from build123d import *

# Parameters (mm, degrees)
F0_W     = 76.2
F0_H     = 19.05
F0_W_2   = 19.05
F0_H_2   = 38.1
F0_R     = 17.4625
F0_W_3   = 20.17304
F1_DEPTH = 19.05
F0_R_2   = 6.35
F2_DEPTH = 9.525


with BuildPart() as f1:
    # F0 (on Front) → F1 (new body)
    with BuildSketch(Plane.XZ):
        Polygon((-489.430563, 76.2), (-540.230563, 76.2), (-540.230563, 95.25), (-591.030563, 95.25), (-599.913724, 95.25), (-613.971884, 125.397822), (-596.706721, 133.4487), (-618.175729, 179.489136), (-635.440892, 171.438258), (-656.9099, 217.478693), (-639.644736, 225.529571), (-661.113744, 271.570007), (-678.378907, 263.519129), (-699.847915, 309.559564), (-682.582752, 317.610442), (-704.051759, 363.650878), (-721.316923, 355.6), (-743.430563, 355.6), (-997.430563, 127), (-997.430563, 0), (-591.030563, 0), (342.419437, 0), (371.914191, 0), (392.43009, 43.996488), (447.893046, 162.937181), (502.200551, 162.937181), (676.493046, 162.937181), (676.493046, 239.137181), (676.493046, 258.187181), (624.570006, 258.187181), (624.570006, 239.137181), (573.770006, 239.137181), (573.770006, 258.187181), (522.970006, 258.187181), (522.970006, 239.137181), (472.170006, 239.137181), (472.170006, 258.187181), (421.370006, 258.187181), (421.370006, 239.137181), (399.256366, 239.137181), (381.991203, 247.188059), (360.522195, 201.147623), (377.787358, 193.096745), (356.318351, 147.05631), (339.053221, 155.107172), (317.579072, 109.055711), (334.844236, 101.004833), (323.369437, 76.2), (272.569437, 76.2), (272.569437, 95.25), (221.769437, 95.25), (221.769437, 76.2), (170.969437, 76.2), (170.969437, 95.25), (120.169437, 95.25), (120.169437, 76.2), (69.369437, 76.2), (69.369437, 95.25), (18.569437, 95.25), (18.569437, 76.2), (-32.230563, 76.2), (-32.230563, 95.25), (-83.030563, 95.25), (-83.030563, 76.2), (-133.830563, 76.2), (-133.830563, 95.25), (-184.630563, 95.25), (-184.630563, 76.2), (-235.430563, 76.2), (-235.430563, 95.25), (-286.230563, 95.25), (-286.230563, 76.2), (-337.030563, 76.2), (-337.030563, 95.25), (-387.830563, 95.25), (-387.830563, 76.2), (-438.630563, 76.2), (-438.630563, 95.25), (-489.430563, 95.25), align=None)
        with Locations((-705.330563, 34.925)):
            Rectangle(F0_W, F0_H, mode=Mode.SUBTRACT)
        with Locations((-581.505563, 44.45)):
            Rectangle(F0_W_2, F0_H_2, mode=Mode.SUBTRACT)
        with Locations((-932.085752, 57.15)):
            Circle(F0_R, mode=Mode.SUBTRACT)
        with Locations((-159.243268, 44.45)):
            Rectangle(F0_W_2, F0_H_2, mode=Mode.SUBTRACT)
        with Locations((351.944437, 44.45)):
            Rectangle(F0_W_2, F0_H_2, mode=Mode.SUBTRACT)
        Polygon((-832.288567, 215.839342), (-845.030563, 230.0007), (-788.385133, 280.968682), (-775.643137, 266.807325), align=None, mode=Mode.SUBTRACT)
        with Locations((411.845006, 201.037181)):
            Rectangle(F0_W_2, F0_H_2, mode=Mode.SUBTRACT)
        with Locations((549.493046, 191.512181)):
            Rectangle(F0_W, F0_H, mode=Mode.SUBTRACT)
        with Locations((641.006526, 201.037181)):
            Rectangle(F0_W_3, F0_H_2, mode=Mode.SUBTRACT)
    extrude(amount=-F1_DEPTH)

    # F0 (on Front) → F2 (join)
    with BuildSketch(Plane.XZ):
        with Locations((-932.085752, 57.15)):
            Circle(F0_R)
        with Locations((-932.085752, 57.15)):
            Circle(F0_R_2, mode=Mode.SUBTRACT)
    extrude(amount=-F2_DEPTH)


solid = f1.part
Part model, mm, in its own coordinate system. A direction names the side the tool comes from. Round coordinates to 2 decimals unless told otherwise and drop trailing zeros. Loops run counter-clockwise (first coordinate to the right, second up) from the corner with the lowest first, then second, coordinate; pieces in that order, holes last. Notation, with made-up numbers: (-27.5, 32.25) - (-12.5, 32.25) arc R10 ccw to (-12.5, 40.25) - close; hole circle Ø11 at (62.25, 17.25). An arc over 180 degrees is marked (long way). Answer as a JSON object with one key per item and string values.
Item 1: Pin check, flat tips, straight feed: pin 1 (5.5 mm diameter, centred on y = 7.5, z = 86.5, fed in from +X); pin 2 (9.5 mm diameter, centred on x = -113, y = 9.5, fed in from +Z); pin 3 (9.5 mm diameter, centred on y = 11.5, z = 83.5, fed in from +X); pin 4 (7.5 mm diameter, centred on x = -932.09, z = 57.15, fed in from -Y). Stop position of each tip, or through.
Output:
{"pin 1": "x = 413.53", "pin 2": "z = 76.2", "pin 3": "x = 413.07", "pin 4": "through"}
Item 2: Tool access for faces 1 (the face through (-949.53, 14.22, 57.92)), 2 (the face through (-350, 19.05, 61)), 3 (the face through (-803.57, 9.39, 241.68)): list every direction of +Z, -Z, +X, -X, +Y, -Y with a clear straight run to the whole face (end or side of a thin tool).
Output:
{"face 1": "+Y", "face 2": "+Z, -Z, +X, -X, +Y", "face 3": "+Y, -Y"}
Item 3: Band-saw the part on A-A on y = 3. State how many separate pieces and enclosed holes the cut face has, plus the area to 3 significant figures.
Output:
{"separate pieces": "1", "enclosed holes": "9", "area": "210,000 mm2"}
Item 4: Wall check: L1, parallel to X at y = 16, z = 42.5; L2, parallel to X at y = 18.75, z = 226; L3, parallel to X at y = 10.75, z = 214. Give the ranges that are in metal, low to high.
Output:
{"L1": "-997.43 to -941.59, -922.58 to -743.43, -667.23 to -591.03, -571.98 to -168.77, -149.72 to 342.42, 361.47 to 391.73", "L2": "-887.43 to -841.43, -821 to -639.86, 372.11 to 676.49", "L3": "-900.76 to -655.29, 366.52 to 402.32, 421.37 to 630.92, 651.09 to 676.49"}
Item 5: Band-saw the part on B-B on x = -558. List the corners of the cut face in (y, z), plus the area to 3 significant figures.
Output:
{"outline": "(0, 0) - (19.05, 0) - (19.05, 95.25) - (0, 95.25) - close", "area": "1,810 mm2"}
Item 6: Pull direction X, two halves, no side cores. Call faces 4 (the face through (-358, 0, 63)), 5 (the face through (-868.65, 9.39, 242.9)), 6 (the face through (-817.1, 9.39, 255.13)): pulls with the +X half, pulls with the -X half, needs draft (parallel to the pull), parting line crosses it, or undercut.
Output:
{"face 4": "needs draft", "face 5": "pulls with the -X half", "face 6": "undercut"}
